The model under review builds one solid part; all positions refer to its coordinate system, in mm. Face numbers are marked on the shaded views. A direction names the side the tool comes from. Coordinates: 2 decimals unless noted, no trailing zeros. Loops run counter-clockwise (first coordinate to the right, second up) from the corner with the lowest first, then second, coordinate; pieces in that order, holes last. Notation, with made-up numbers: (24, 9.5) - (56, 9.5) arc R24 cw to (56, 28.5) - close; hole circle Ø9 at (10.25, 17.25). An arc over 180 degrees is marked (long way). One line per item, written item: value. Start each with the question number.
1. We need section D-D, the plane z = -23. Give the boundary of the cut face in (x, y), then the cut area to 3 significant figures.
2. Insertion check: P1, Ø1.5, axis at x = 3, z = -24, coming from the -Y side; P2, Ø2, axis at x = -2.5, y = 1, coming from the +Z side; P3, Ø0.8, axis at x = -6, y = -1, coming from the -Z side. Each pin has a flat end and moves straight along its axis. Give the tip position at first contact, or say it passes through.
3. We need section B-B, the plane z = 1. Give the boundary of the cut face in (x, y).
4. To check wall thickness, follow line 1 (Y direction, x = 2.25, z = -7.5); line 2 (Z direction, x = 4.5, y = 0.5); line 3 (X direction, y = 1.75, z = 3). State the ranges of each line that lie inside material, in increasing order.
5. For the marked faces 1, 2, 3, 4 and 5, list the 3-axis set-ups (+Z, -Z, +X, -X, +Y, -Y) from which the entire face can be reached by the end or side of a thin tool; tool diameter is ignored.
6. We need section A-A, the plane y = -3.05. Give the boundary of the cut face in (x, z).
7. We need section C-C, the plane x = -2.5. Give the boundary of the cut face in (y, z).
from build123d import *

# Parameters (mm, degrees)
EXTRUDE_1_DEPTH          = 2
EXTRUDE_START            = -8
EXTRUDE_2_DEPTH          = 8
CUT_EXTRUDE_1_DEPTH      = 23.468559083
CUT_EXTRUDE_1_DEPTH_BACK = 23.468559083
EXTRUDE_3_DEPTH          = 5.5
CUT_EXTRUDE_START        = 1.7
SKETCH_6_OUTSIDE_W       = 26.07
SKETCH_6_OUTSIDE_H       = 16.37
CUT_EXTRUDE_2_DEPTH      = 19.782223


with BuildPart() as part:
    # 草图1 → 凸台-拉伸1 (new body)
    with BuildSketch(Plane(origin=(0, 0, 0), x_dir=(1, 0, 0), z_dir=(0, 1, 0))):
        with BuildLine():
            Line((-7.6, -2.497999199), (-7.6, 7.9206403))
            ThreePointArc((-7.6, 7.9206403), (0, 9.5), (7.6, 7.9206403))
            Line((7.6, 7.9206403), (7.6, -2.497999199))
            ThreePointArc((7.6, -2.497999199), (0, -8), (-7.6, -2.497999199))
        make_face()
        Polygon((0, 5.411961001), (-3.826834324, 3.826834324), (-5.411961001, 0), (-3.826834324, -3.826834324), (0, -5.411961001), (3.826834324, -3.826834324), (5.411961001, 0), (3.826834324, 3.826834324), align=None, mode=Mode.SUBTRACT)
    extrude(amount=EXTRUDE_1_DEPTH)

    # 草图3 → 凸台-拉伸2 (add)
    with BuildSketch(Plane(origin=(0, 2, 0), x_dir=(1, 0, 0), z_dir=(0, 1, 0)).offset(EXTRUDE_START)):
        with BuildLine():
            Line((-7.6, 7.9206403), (-7.6, 15.4206403))
            Line((-7.6, 15.4206403), (0, 13.517776718))
            Line((0, 13.517776718), (7.6, 15.4206403))
            Line((7.6, 15.4206403), (7.6, 7.9206403))
            ThreePointArc((7.6, 7.9206403), (0, 9.5), (-7.6, 7.9206403))
        make_face()
    extrude(amount=EXTRUDE_2_DEPTH)

    # 草图4 → 切除-拉伸1 (cut, two sides: drawn at the far end of the back side and taken through both)
    with BuildSketch(Plane(origin=(7.6, 0, 0), x_dir=(0, 0, -1), z_dir=(1, 0, 0)).offset(-CUT_EXTRUDE_1_DEPTH_BACK)):
        Polygon((15.4206403, 2), (8.364338974, 2), (15.4206403, -1.292940619), align=None)
        Polygon((15.4206403, -6), (15.4206403, -3.5), (7.9206403, 0), (7.9206403, -6), align=None)
    extrude(amount=CUT_EXTRUDE_1_DEPTH + CUT_EXTRUDE_1_DEPTH_BACK, mode=Mode.SUBTRACT)

    # 草图5 → 凸台-拉伸3 (add)
    with BuildSketch(Plane(origin=(0, 2, 0), x_dir=(1, 0, 0), z_dir=(0, 1, 0))):
        with BuildLine():
            Line((-7.6, 15.4206403), (-7.6, 27.797999199))
            ThreePointArc((-7.6, 27.797999199), (0, 33.3), (7.6, 27.797999199))
            Line((7.6, 27.797999199), (7.6, 15.4206403))
            Line((7.6, 15.4206403), (0, 13.517776718))
            Line((0, 13.517776718), (-7.6, 15.4206403))
        make_face()
    extrude(amount=-EXTRUDE_3_DEPTH)

    # 草图6 outside → 切除-拉伸2 (cut)
    with BuildSketch(Plane.XY.offset(-35).offset(CUT_EXTRUDE_START)):
        with Locations((0, -0.75)):
            Rectangle(SKETCH_6_OUTSIDE_W, SKETCH_6_OUTSIDE_H)
        with BuildLine():
            Line((7.6, -1.446364095), (1.062655153, 0.077764377))
            ThreePointArc((1.062655153, 0.077764377), (0, 0.2), (-1.062655153, 0.077764377))
            Line((-1.062655153, 0.077764377), (-7.6, -1.446364095))
            Line((-7.6, -1.446364095), (-7.6, -3.5))
            Line((-7.6, -3.5), (-0.608549693, -1.870000556))
            ThreePointArc((-0.608549693, -1.870000556), (0, -1.8), (0.608549693, -1.870000556))
            Line((0.608549693, -1.870000556), (7.6, -3.5))
            Line((7.6, -3.5), (7.6, -1.446364095))
        make_face(mode=Mode.SUBTRACT)
    extrude(amount=CUT_EXTRUDE_2_DEPTH, mode=Mode.SUBTRACT)


solid = part.part
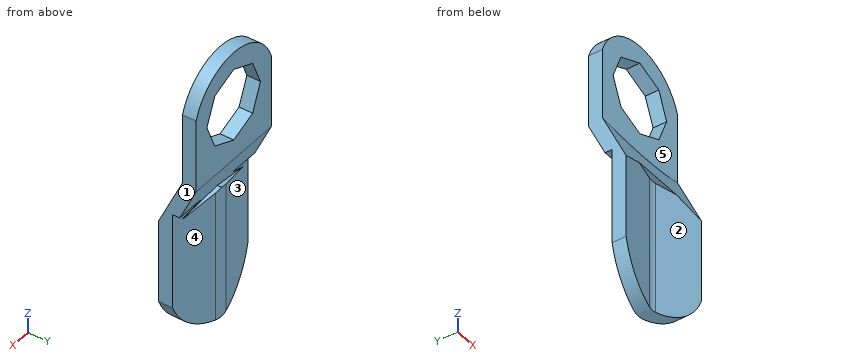
Findings below:
1. outline: (-7.6, -3.5) - (-0.61, -1.87) arc R2.68 cw to (0.61, -1.87) - (7.6, -3.5) - (7.6, -1.45) - (1.06, 0.08) arc R4.68 ccw to (-1.06, 0.08) - (-7.6, -1.45) - close
1. area: 31.2 mm2
2. P1: y = -2.6
2. P2: z = 7.86
2. P3: z = -31.01
3. outline: (-7.6, 0) - (-5, 0) - (-5, 2) - (-7.6, 2) - close; (5, 0) - (7.6, 0) - (7.6, 2) - (5, 2) - close
4. line 1: 0 to 2
4. line 2: -11.58 to -2.2, 2.2 to 6.61
4. line 3: -7.42 to -4.17, 4.17 to 7.42
5. face 1: +Z, -Z, +X, +Y, -Y
5. face 2: -Z, -Y
5. face 3: -Z, -X, +Y
5. face 4: -Z, +X, +Y
5. face 5: +Z, -Y
6. outline: (-7.6, -27.8) arc R8 ccw to (-5.67, -30.94) - (-5.67, -14.46) - (-7.6, -14.46) - close; (5.67, -30.94) arc R8 ccw to (7.6, -27.8) - (7.6, -14.46) - (5.67, -14.46) - close
7. outline: (-2.61, -13.52) - (-2.31, -13.52) - (-2.31, -32.9) - (-0.26, -32.9) - (-0.26, -14.14) - (-0.7, -14.14) - (2, -8.36) - (2, -4.38) - (0, -4.38) - (0, -9.34) - (-0.66, -9.34) - close; (0, 4.38) - (2, 4.38) - (2, 7.6) - (0, 7.6) - close
